Here's the drawing with two shaded views (mm, measured from the low corner). I have some questions. A direction names the side the tool comes from. Give positions to 0.01 mm unless a question says otherwise; leave off trailing zeros. Write each loop counter-clockwise with the first axis right and the second up, starting at its lowest first coordinate (ties: lowest second). Pieces come first, ordered by that corner, then holes. Notation, with made-up numbers: (-39, -24) -> (-30, -24) arc R16 ccw to (-30, 0) -> close; hole circle Ø10 at (9, 83). An arc over 180 degrees is marked (long way). One line per item, written item: value.
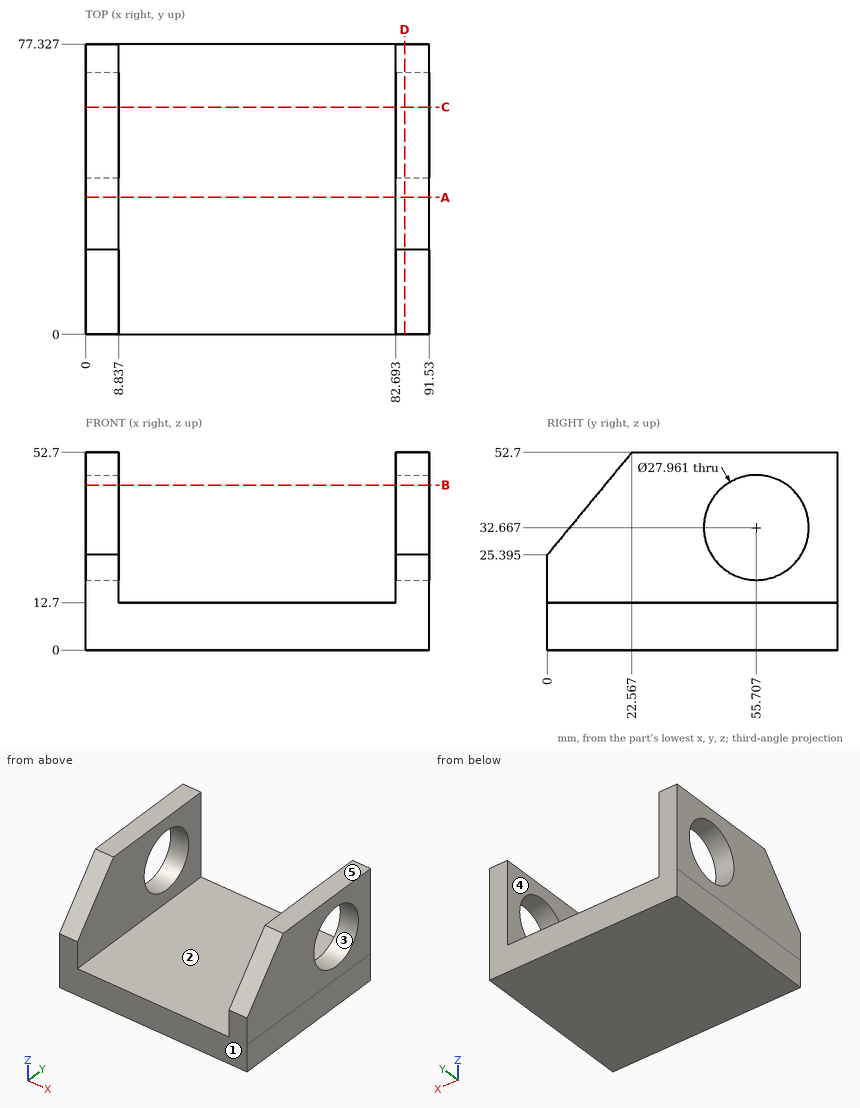
1) I need wall thicknesses on L1, parallel to X at y = 16.5, z = 43; L2, parallel to Z at x = 51, y = 54.5; L3, parallel to Y at x = 4, z = 40.5 (1 decimal). Which ranges of each line are inside material? Lowest first, please.
Answer list:
L1: x = 0 to 8.84, 82.69 to 91.53
L2: z = 0 to 12.7
L3: y = 12.5 to 44.1, 67.3 to 77.3
2) We'd pull the mould along Z, two halves only. Please class the marked faces 3, 4 and 5: released by +Z, released by -Z, zero draft, split by the parting line, or undercut.
Answer list:
face 3: undercut
face 4: zero draft
face 5: released by +Z
3) Will these pins go through, and if not, where does the flat tip stop? pin 1 (12 mm diameter, centred on y = 51.5, z = 32, fed in from +X); pin 2 (5 mm diameter, centred on x = 31.5, y = 27.5, fed in from -Z); pin 3 (1.5 mm diameter, centred on x = 49, y = 43, fed in from +Z).
Answer list:
pin 1: passes through
pin 2: stops at z = 0
pin 3: stops at z = 12.7
4) If we section it at D-D (x = 85): Write out the boundary of the cut face in (y, z) (1 decimal), and give its area (3 significant figures).
Answer list:
outline: (0, 0) -> (77.3, 0) -> (77.3, 52.7) -> (22.6, 52.7) -> (0, 25.4) -> close; hole circle Ø28 at (55.7, 32.7)
area: 3,150 mm^2
5) If we section it at C-C (y = 60.5): Write out the boundary of the cut face in (x, z), and give its area (4 significant figures).
Answer list:
outline: (0, 0) -> (91.53, 0) -> (91.53, 19.53) -> (82.69, 19.53) -> (82.69, 12.7) -> (8.84, 12.7) -> (8.84, 19.53) -> (0, 19.53) -> close; (0, 45.8) -> (8.84, 45.8) -> (8.84, 52.7) -> (0, 52.7) -> close; (82.69, 45.8) -> (91.53, 45.8) -> (91.53, 52.7) -> (82.69, 52.7) -> close
area: 1,405 mm^2
6) If we section it at A-A (y = 36.5): Write out the boundary of the cut face in (x, z).
Answer list:
outline: (0, 0) -> (91.53, 0) -> (91.53, 52.7) -> (82.69, 52.7) -> (82.69, 12.7) -> (8.84, 12.7) -> (8.84, 52.7) -> (0, 52.7) -> close
7) For the marked faces 1 and 2, which set-ups out of +Z, -Z, +X, -X, +Y, -Y let a thin tool reach every point of the face, with its end or its side?
Answer list:
face 1: +Z, -Z, +X, -X, -Y
face 2: +Z, +Y, -Y
8) If we section it at B-B (z = 44): Write out the boundary of the cut face in (x, y).
Answer list:
outline: (0, 15.38) -> (8.84, 15.38) -> (8.84, 47.52) -> (0, 47.52) -> close; (0, 63.89) -> (8.84, 63.89) -> (8.84, 77.33) -> (0, 77.33) -> close; (82.69, 15.38) -> (91.53, 15.38) -> (91.53, 47.52) -> (82.69, 47.52) -> close; (82.69, 63.89) -> (91.53, 63.89) -> (91.53, 77.33) -> (82.69, 77.33) -> close
